Autodesk Inventor part; units mm, degrees
ref_plane "YZ Plane" through (0, 0, 0) normal (1, 0, 0) x (0, 1, 0)
ref_plane "XZ Plane" through (0, 0, 0) normal (0, 1, 0) x (-1, 0, 0)
ref_plane "XY Plane" through (0, 0, 0) normal (0, 0, 1) x (1, 0, 0)
sketch "Sketch1" plane through (0, 0, 0) normal (0, 0, 1) x (1, 0, 0)
  line L0 (0, 0) -> (25.4, 0)
  line L1 (25.4, 0) -> (25.4, 3.175)
  line L2 (3.175, 50.8) -> (0, 50.8)
  line L3 (0, 50.8) -> (0, 0)
  line L4 (3.175, 50.8) -> (3.175, 3.175)
  line L5 (3.175, 3.175) -> (25.4, 3.175)
  dimension "d0" = 50.8
  dimension "d1" = 25.4
  dimension "d2" = 3.175
extrude "Extrusion1" add sketch "Sketch1" along normal blind 76.2
sketch "Sketch2" plane through (0, 0, 0) normal (-1, 0, 0) x (0, 0, 1)
  line L0 (76.2, 0) -> (76.2, 50.8)
  line L1 (0, 50.8) -> (76.2, 50.8)
  line L2 (0, 50.8) -> (0, 0)
  line L3 (0, 0) -> (76.2, 0)
  line L4 (50.8, 50.8) -> (50.8, 0) construction
  line L5 (50.8, 50.8) -> (0, 3.175)
  dimension "d5" = 25.4
  dimension "d6" = 3.175
extrude "Extrusion2" cut sketch "Sketch2" against normal blind 25.4 contours L5 L2 L1
properties part number "manipulator corner brace right"
For this review, take the finished solid that the model builds, in its own axes (mm). A direction names the side the tool comes from. Coordinates: 2 decimals unless noted, no trailing zeros. Order: outer loops, then holes, each group sorted by start corner. A loop starts at its lowest first (then second) coordinate and runs counter-clockwise, first axis right, second up. Notation, with made-up numbers: (-12, -16) - (-6, -16) arc R16 ccw to (-6, -9) - close; hole circle Ø1 at (1, 74.25). An arc over 180 degrees is marked (long way). Answer as a JSON object with one key per item and string values. Group by question number.
1. We need section A-A on z = 56. State the section outline as (x, y) points (3 decimals), then the cut area to 3 significant figures.
2. We need section B-B on y = 10. State the section outline as (x, z) points (3 decimals), then the cut area to 3 significant figures.
3. We need section D-D on z = 6. State the section outline as (x, y) points (3 decimals).
4. The part is to be moulded in two halves that separate along Z. For faces 3 (the flat face through (1.565, 27.321, 25.756)), 4 (the flat face through (2, 18, 76.2)), 5 (the flat face through (25.4, 2, 38)), say which applies: pulls with the +Z half, pulls with the -Z half, needs draft (parallel to the pull), parting line crosses it, or undercut.
5. Clearance check with flat-ended pins moving along their axes: P1, Ø1, axis at y = 31, z = 42.5, coming from the +X side (3 decimals); P2, Ø6, axis at x = 9, y = 25.5, coming from the +Z side; P3, Ø12, axis at x = 14.5, z = 21.5, coming from the +Y side (3 decimals). State where each tip first meets the part, or that it passes through.
6. We need section C-C on x = 12.25. State the section outline as (y, z) points (3 decimals).
7. For faces 1 (the flat face through (13, 0, 38)), 2 (the flat face through (14, 3.175, 38)), list the 3-axis set-ups (+Z, -Z, +X, -X, +Y, -Y) from which the entire face can be reached by the end or side of a thin tool; tool diameter is ignored.
8. For probe 1 along Y at (x, z) = (4.5, 62.5) (3 decimals); probe 2 along Y at (x, z) = (1.75, 46), list the stretches that pass through material, from the lowest coordinate up.
Final values:
{
 "1": {"outline": "(0, 0) - (25.4, 0) - (25.4, 3.175) - (3.175, 3.175) - (3.175, 50.8) - (0, 50.8) - close", "area": "232 mm²"},
 "2": {"outline": "(0, 7.28) - (3.175, 7.28) - (3.175, 76.2) - (0, 76.2) - close", "area": "219 mm²"},
 "3": {"outline": "(0, 0) - (25.4, 0) - (25.4, 3.175) - (3.175, 3.175) - (3.175, 8.8) - (0, 8.8) - close"},
 "4": {"face 3": "pulls with the -Z half", "face 4": "pulls with the +Z half", "face 5": "needs draft"},
 "5": {"P1": "x = 3.175", "P2": "through", "P3": "y = 3.175"},
 "6": {"outline": "(0, 0) - (3.175, 0) - (3.175, 76.2) - (0, 76.2) - close"},
 "7": {"face 1": "+Z, -Z, +X, -X, -Y", "face 2": "+Z, -Z, +X, +Y"},
 "8": {"probe 1": "0 to 3.175", "probe 2": "0 to 46.3"}
}
